Here's how the part is built. I have some questions about the finished solid (model axes, mm). Coordinates: 2 decimals unless noted, no trailing zeros. Write each loop counter-clockwise with the first axis right and the second up, starting at its lowest first coordinate (ties: lowest second). Pieces come first, ordered by that corner, then holes. Notation, with made-up numbers: (77, -15) - (100, -15) arc R19 cw to (100, 17) - close; hole circle Ø7 at (16.25, 48). An arc over 180 degrees is marked (long way). Answer in a Markdown table with one row per item. Add a question column.
Item 1: I'm going to push a flat-ended pin straight in: pin 1 (1 mm diameter, centred on x = 8.5, y = 4, fed in from +Z). Where does the tip first touch, or does it pass through?
Item 2: If I drill on probe 1 along Z at (x, y) = (14, 3); probe 2 along Y at (x, z) = (10.75, -1.95); probe 3 along Y at (x, z) = (6.75, -2), over which ranges is the centre line in solid material (lowest first)? Write a range as from..to.
Item 3: Imagine slicing it at B-B (x = 6.25). Please give me the cut outline in (y, z), plus the area to 3 significant figures.
Item 4: Imagine slicing it at A-A (y = 7). Please give me the cut outline in (x, z).
from build123d import *

# Parameters (mm, degrees)
SKETCH1_W                  = 15.24
SKETCH1_H                  = 3.556
BOSS_EXTRUDE1_DEPTH        = 8.636
SKETCH2_W                  = 0.635
SKETCH2_H                  = 0.635
CUT_EXTRUDE1_DEPTH         = 6.35
CHAMFER1_SIZE              = 0.508
LPATTERN1_COUNT            = 6
LPATTERN1_PITCH            = 2.54
CHAMFER1_OF_LPATTERN1_SIZE = 0.508


with BuildPart() as part:
    # Sketch1 → Boss-Extrude1 (new body)
    with BuildSketch(Plane(origin=(0, 0, 0), x_dir=(1, 0, 0), z_dir=(0, 1, 0))):
        with Locations((7.62, 1.778)):
            Rectangle(SKETCH1_W, SKETCH1_H)
    extrude(amount=BOSS_EXTRUDE1_DEPTH)

    # Sketch2 → Cut-Extrude1 (cut)
    with BuildSketch(Plane(origin=(0, 8.636, 0), x_dir=(1, 0, 0), z_dir=(0, 1, 0))):
        with Locations((1.27, 1.778)):
            Rectangle(SKETCH2_W, SKETCH2_H)
    cut_extrude1 = extrude(amount=-CUT_EXTRUDE1_DEPTH, mode=Mode.SUBTRACT)

    # Chamfer1
    chamfer1_edges = [part.edges().sort_by_distance(p)[0] for p in [
        (1.5875, 8.636, -1.778),
        (1.27, 8.636, -2.0955),
        (0.9525, 8.636, -1.778),
        (1.27, 8.636, -1.4605),
    ]]
    chamfer(chamfer1_edges, length=CHAMFER1_SIZE)

    # LPattern1: Cut-Extrude1 ×6
    with Locations(*[(i * LPATTERN1_PITCH, 0, 0) for i in range(1, LPATTERN1_COUNT)]):
        add(cut_extrude1, mode=Mode.SUBTRACT)

    # Chamfer1 of LPattern1
    chamfer1_of_lpattern1_edges = [part.edges().sort_by_distance(p)[0] for p in [
        (4.1275, 8.636, -1.778),
        (3.81, 8.636, -2.0955),
        (3.4925, 8.636, -1.778),
        (3.81, 8.636, -1.4605),
        (6.6675, 8.636, -1.778),
        (6.35, 8.636, -2.0955),
        (6.0325, 8.636, -1.778),
        (6.35, 8.636, -1.4605),
        (9.2075, 8.636, -1.778),
        (8.89, 8.636, -2.0955),
        (8.5725, 8.636, -1.778),
        (8.89, 8.636, -1.4605),
        (11.7475, 8.636, -1.778),
        (11.43, 8.636, -2.0955),
        (11.1125, 8.636, -1.778),
        (11.43, 8.636, -1.4605),
        (14.2875, 8.636, -1.778),
        (13.97, 8.636, -2.0955),
        (13.6525, 8.636, -1.778),
        (13.97, 8.636, -1.4605),
    ]]
    chamfer(chamfer1_of_lpattern1_edges, length=CHAMFER1_OF_LPATTERN1_SIZE)


solid = part.part
Here are the results:
| question | item | result |
|---|---|---|
| 1 | pin 1 | stops at z = 0 |
| 2 | probe 1 | z = -3.56..-2.1, -1.46..0 |
| 2 | probe 2 | y = 0..8.49 |
| 2 | probe 3 | y = 0..8.21 |
| 3 | outline | (0, -3.56) - (8.64, -3.56) - (8.64, -2.6) - (8.13, -2.1) - (2.29, -2.1) - (2.29, -1.46) - (8.13, -1.46) - (8.64, -0.95) - (8.64, 0) - (0, 0) - close |
| 3 | area | 26.4 mm2 |
| 4 | outline | (0, -3.56) - (15.24, -3.56) - (15.24, 0) - (0, 0) - close; hole (0.95, -2.1) - (1.59, -2.1) - (1.59, -1.46) - (0.95, -1.46) - close; hole (3.49, -2.1) - (4.13, -2.1) - (4.13, -1.46) - (3.49, -1.46) - close; hole (6.03, -2.1) - (6.67, -2.1) - (6.67, -1.46) - (6.03, -1.46) - close; hole (8.57, -2.1) - (9.21, -2.1) - (9.21, -1.46) - (8.57, -1.46) - close; hole (11.11, -2.1) - (11.75, -2.1) - (11.75, -1.46) - (11.11, -1.46) - close; hole (13.65, -2.1) - (14.29, -2.1) - (14.29, -1.46) - (13.65, -1.46) - close |
